Work out the finished part from the listing and answer in its coordinate system (mm). A direction names the side the tool comes from. Round coordinates to 2 decimals unless told otherwise and drop trailing zeros. Write each loop counter-clockwise with the first axis right and the second up, starting at its lowest first coordinate (ties: lowest second). Pieces come first, ordered by that corner, then holes. Notation, with made-up numbers: (-4, 70) - (6, 70) arc R23 cw to (6, 100) - close; hole circle Ø4 at (14, -29.5). An arc over 180 degrees is marked (long way). Answer as a JSON object with one key per item and string values.
```python
from build123d import *

# Parameters (mm, degrees)
PAD001_DEPTH    = 22
SKETCH005_R     = 1.65
POCKET003_DEPTH = 24.001
SKETCH006_R     = 2.75
POCKET004_DEPTH = 16.001
SKETCH007_R     = 3.25
POCKET005_DEPTH = 61.001
SKETCH008_R     = 5.75
POCKET006_DEPTH = 11


with BuildPart() as part:
    # Sketch004 → Pad001 (new body)
    with BuildSketch(Plane.XZ.offset(11)):
        with BuildLine():
            Line((-20.1, 5), (-19.1, 10))
            Line((-9.5, 14.5), (-19.1, 10))
            ThreePointArc((9.5, 14.5), (0, 24), (-9.5, 14.5))
            Line((9.5, 14.5), (19.1, 10))
            Line((20.1, 5), (19.1, 10))
            Line((9.5, 5), (20.1, 5))
            Line((9.5, 5), (6.717514, 7.782486))
            ThreePointArc((-6.717514, 7.782486), (0, 5), (6.717514, 7.782486))
            Line((-9.5, 5), (-6.717514, 7.782486))
            Line((-20.1, 5), (-9.5, 5))
        make_face()
    extrude(amount=-PAD001_DEPTH)

    # Sketch005 → Pocket003 (cut, through all)
    with BuildSketch(Plane.XY):
        with Locations((-15.5, 7.5)):
            Circle(SKETCH005_R)
        with Locations((15.5, 7.5)):
            Circle(SKETCH005_R)
        with Locations((15.5, -7.5)):
            Circle(SKETCH005_R)
        with Locations((-15.5, -7.5)):
            Circle(SKETCH005_R)
    extrude(amount=POCKET003_DEPTH, mode=Mode.SUBTRACT)

    # Sketch006 → Pocket004 (cut, through all)
    with BuildSketch(Plane.XY.offset(8)):
        with Locations((-15.5, 7.5)):
            Circle(SKETCH006_R)
        with Locations((-15.5, -7.5)):
            Circle(SKETCH006_R)
        with Locations((15.5, 7.5)):
            Circle(SKETCH006_R)
        with Locations((15.5, -7.5)):
            Circle(SKETCH006_R)
    extrude(amount=POCKET004_DEPTH, mode=Mode.SUBTRACT)

    # Sketch007 → Pocket005 (cut, through all)
    with BuildSketch(Plane.XZ.offset(50)):
        with Locations((0, 14.5)):
            Circle(SKETCH007_R)
    extrude(amount=-POCKET005_DEPTH, mode=Mode.SUBTRACT)

    # Sketch008 → Pocket006 (cut)
    with BuildSketch(Plane.XZ.offset(11)):
        with Locations((0, 14.5)):
            Circle(SKETCH008_R)
    extrude(amount=-POCKET006_DEPTH, mode=Mode.SUBTRACT)


solid = part.part
```
Item 1: Determine the mould class of faces 4 (the cylindrical face through (17.024, -8.132, 6.479)), 5 (the flat face through (17, -9, 8)), 6 (the flat face through (0, -11, 8)), 7 (the flat face through (19.6, -0.2, 7.5)) for opening direction Y: pulls with the +Y half, pulls with the -Y half, needs draft (parallel to the pull), parting line crosses it, or undercut.
Results found:
{"face 4": "undercut", "face 5": "undercut", "face 6": "pulls with the -Y half", "face 7": "needs draft"}
Item 2: For faces 1 (the cylindrical face through (-4.56, -5.58, 11)), 2 (the flat face through (8.1, -0.2, 6.4)), 3 (the cylindrical face through (-12.96, -8.55, 9.9)), determine the directions among +Z, -Z, +X, -X, +Y, -Y from which every point of the face is accessible in a straight line to the end or side of a thin tool.
Results found:
{"face 1": "-Y", "face 2": "-Z, +Y, -Y", "face 3": "+Z"}
Item 3: A cutting plane is placed at D-D (x = 15.5). Write down the section's boundary in (y, z), and give its area (3 significant figures).
Results found:
{"outline": "(-11, 5) - (-9.15, 5) - (-9.15, 8) - (-10.25, 8) - (-10.25, 11.69) - (-11, 11.69) - close; (-5.85, 5) - (5.85, 5) - (5.85, 8) - (4.75, 8) - (4.75, 11.69) - (-4.75, 11.69) - (-4.75, 8) - (-5.85, 8) - close; (9.15, 5) - (11, 5) - (11, 11.69) - (10.25, 11.69) - (10.25, 8) - (9.15, 8) - close", "area": "86.8 mm²"}
Item 4: A cutting plane is placed at C-C (z = 16). Write down the section's boundary in (x, y), and give its area (3 significant figures).
Results found:
{"outline": "(-9.38, -11) - (-5.55, -11) - (-5.55, 0) - (-2.88, 0) - (-2.88, 11) - (-9.38, 11) - close; (2.88, 0) - (5.55, 0) - (5.55, -11) - (9.38, -11) - (9.38, 11) - (2.88, 11) - close", "area": "227 mm²"}
Item 5: Each of these flat-tipped pins is pushed along its axis until it touches: P1, Ø6.5, axis at x = 15.5, y = 7.5, coming from the +Z side; P2, Ø4.5, axis at x = 15.5, y = 7.5, coming from the +Z side; P3, Ø3, axis at x = 15.5, y = -7.5, coming from the -Z side; P4, Ø9, axis at x = -15.5, y = 7.5, coming from the +Z side. Where does it stop, or does it pass through?
Results found:
{"P1": "z = 13.21", "P2": "z = 8", "P3": "through", "P4": "z = 13.8"}
Item 6: A cutting plane is placed at A-A (y = -7.5). Write down the section's boundary in (x, z), and give its area (3 significant figures).
Results found:
{"outline": "(-20.1, 5) - (-17.15, 5) - (-17.15, 8) - (-18.25, 8) - (-18.25, 10.4) - (-19.1, 10) - close; (-13.85, 5) - (-9.5, 5) - (-6.72, 7.78) arc R9.5 ccw to (6.72, 7.78) - (9.5, 5) - (13.85, 5) - (13.85, 8) - (12.75, 8) - (12.75, 12.98) - (9.5, 14.5) arc R9.5 ccw to (-9.5, 14.5) - (-12.75, 12.98) - (-12.75, 8) - (-13.85, 8) - close; (17.15, 5) - (20.1, 5) - (19.1, 10) - (18.25, 10.4) - (18.25, 8) - (17.15, 8) - close; hole circle Ø11.5 at (0, 14.5)", "area": "283 mm²"}
Item 7: A cutting plane is placed at B-B (x = 0). Write down the section's boundary in (y, z), and give its area (3 significant figures).
Results found:
{"outline": "(-11, 5) - (11, 5) - (11, 11.25) - (0, 11.25) - (0, 8.75) - (-11, 8.75) - close; (-11, 20.25) - (0, 20.25) - (0, 17.75) - (11, 17.75) - (11, 24) - (-11, 24) - close", "area": "220 mm²"}
Item 8: Consider line 1 along Y through (x, z) = (15.5, 11.05); line 2 along Y through (x, z) = (15.5, 7.2); line 3 along X through (y, z) = (-1.5, 7). Determine where each line is inside the solid, lowest interval first.
Results found:
{"line 1": "-11 to -10.25, -4.75 to 4.75, 10.25 to 11", "line 2": "-11 to -9.15, -5.85 to 5.85, 9.15 to 11", "line 3": "-19.7 to -7.5, -5.83 to 5.83, 7.5 to 19.7"}
